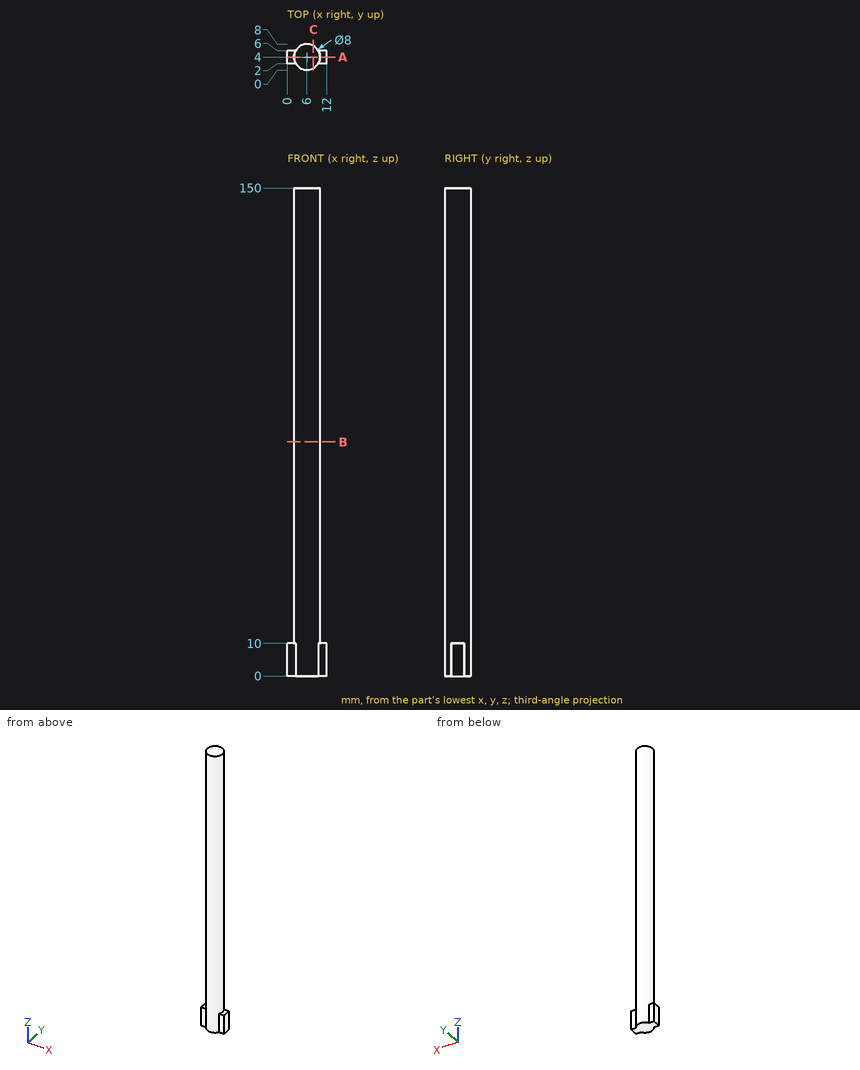
Source: three-view drawing plus pictorial views. Frame: mm from the lowest corner of the part. Round coordinates to 2 decimals unless told otherwise and drop trailing zeros. Loops run counter-clockwise (first coordinate to the right, second up) from the corner with the lowest first, then second, coordinate; pieces in that order, holes last. Notation, with made-up numbers: (46, -33.75) - (50, -33.75) arc R18 ccw to (50, 1.25) - close; hole circle Ø9 at (40, 66.5). An arc over 180 degrees is marked (long way). Write item = value, one per line. Start each with the question number.
Item 1: First-contact query: pin 1 Ø1.3 at (x, z) = (0.5, 5.5) entering from -Y; pin 2 Ø2 at (y, z) = (2, 87) entering from -X; pin 3 Ø4 at (x, z) = (8.5, 93) entering from -Y. Flat tips, straight axial feed; report the tip coordinate or a pass-through.
Item 2: Material intervals for line 1 (X direction, y = 6, z = 122); line 2 (Z direction, x = 11, y = 2.75); line 3 (Y direction, x = 5.75, z = 87), sorted ascending.
Item 3: Section query B-B on z = 72. Output: boundary loops of the cut face in (x, y), plus the area to 3 significant figures.
Item 4: Section query A-A on y = 4. Output: boundary loops of the cut face in (x, z), plus the area to 3 significant figures.
Item 5: Section query C-C on x = 8. Output: boundary loops of the cut face in (y, z), plus the area to 3 significant figures.
Results list:
q1.pin_1 = 2
q1.pin_2 = 2.13
q1.pin_3 = 0.03
q2.line_1 = 2.54 to 9.46
q2.line_2 = 0 to 10
q2.line_3 = 0.01 to 7.99
q3.outline = circle Ø8 at (6, 4)
q3.area = 50.3 mm²
q4.outline = (0, 0) - (12, 0) - (12, 10) - (10, 10) - (10, 150) - (2, 150) - (2, 10) - (0, 10) - close
q4.area = 1,240 mm²
q5.outline = (0.54, 0) - (7.46, 0) - (7.46, 150) - (0.54, 150) - close
q5.area = 1,040 mm²
